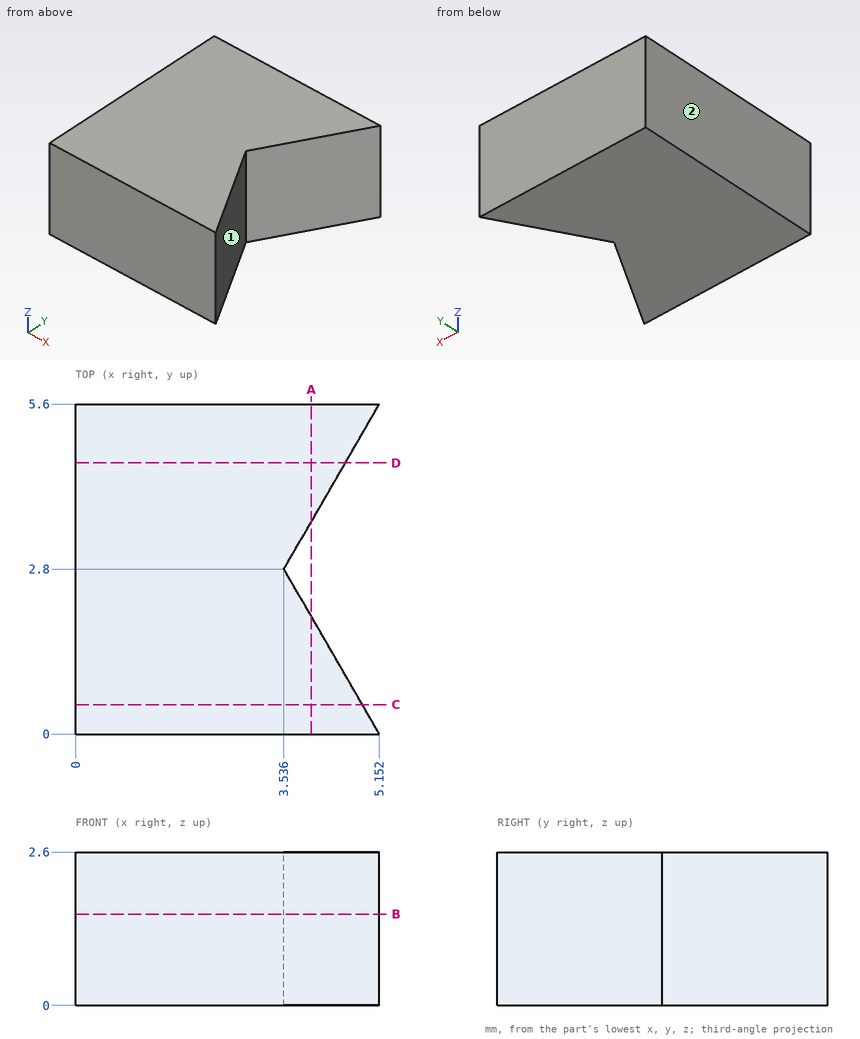
Verification items for this drawing (mm, ordinates from the low corner). A direction names the side the tool comes from. Round coordinates to 2 decimals unless told otherwise and drop trailing zeros. Order: outer loops, then holes, each group sorted by start corner. A loop starts at its lowest first (then second) coordinate and runs counter-clockwise, first axis right, second up. Notation, with made-up numbers: (28, -13) - (36, -13) arc R20 cw to (36, 16) - close; hole circle Ø1 at (29, 69). An arc over 180 degrees is marked (long way). Use CSV: the item, a comma, the result in double quotes. Start each with the question number.
1) Access from +Z, -Z, +X, -X, +Y, -Y to the whole of each face (thin tool, end or side, straight path). Record for the marked faces 1 and 2.
2) Section check C-C, the plane y = 0.5. Record the cut outline in (x, z).
3) Section check A-A, the plane x = 4. Record the cut outline in (y, z), plus the area to 3 significant figures.
4) Section check B-B, the plane z = 1.55. Record the cut outline in (x, y) (1 decimal).
5) Section check D-D, the plane y = 4.6. Record the cut outline in (x, z) (1 decimal), plus the area to 3 significant figures.
6) Thickness scan on L1, parallel to Y at x = 3.6, z = 1.9 (1 decimal); L2, parallel to X at y = 3.2, z = 0.95 (1 decimal); L3, parallel to Y at x = 4.75, z = 0.35 (1 decimal). Record the ranges inside material, lowest first.
Answers:
1,face 1,"+Z, -Z, +X"
1,face 2,"+Z, -Z, -X, +Y, -Y"
2,outline,"(0, 0) - (4.86, 0) - (4.86, 2.6) - (0, 2.6) - close"
3,outline,"(0, 0) - (2, 0) - (2, 2.6) - (0, 2.6) - close; (3.6, 0) - (5.6, 0) - (5.6, 2.6) - (3.6, 2.6) - close"
3,area,"10.4 mm²"
4,outline,"(0, 0) - (5.2, 0) - (3.5, 2.8) - (5.2, 5.6) - (0, 5.6) - close"
5,outline,"(0, 0) - (4.6, 0) - (4.6, 2.6) - (0, 2.6) - close"
5,area,"11.9 mm²"
6,L1,"y = 0 to 2.7, 2.9 to 5.6"
6,L2,"x = 0 to 3.8"
6,L3,"y = 0 to 0.7, 4.9 to 5.6"
